Design review of the part shown in the three views and the two pictorial views. Dimensions are in mm from the part's minimum x, y and z. A direction names the side the tool comes from. Coordinates: 2 decimals unless noted, no trailing zeros. Loops run counter-clockwise (first coordinate to the right, second up) from the corner with the lowest first, then second, coordinate; pieces in that order, holes last. Notation, with made-up numbers: (4.25, -26.5) -> (19.25, -26.5) arc R22 cw to (19.25, 1.5) -> close; hole circle Ø9 at (78, 37.5). An arc over 180 degrees is marked (long way). One line per item, written item: value. Start each with the question number.
1. Add section D-D on y = 3.5. Write out the cut boundary in (x, z).
2. Insertion check: pin 1 (1.1 mm diameter, centred on x = 8.5, z = 1.5, fed in from -Y); pin 2 (4 mm diameter, centred on x = 16, y = 4, fed in from +Z). Each pin has a flat end and moves straight along its axis. Give the tip position at first contact, or say it passes through.
3. For probe 1 along Y at (x, z) = (5.25, 1.75); probe 2 along Z at (x, y) = (12, 3.5); probe 3 along Y at (x, z) = (4.5, 8.75), list the stretches that pass through material, from the lowest coordinate up.
4. Add section A-A on y = 1.75. Write out the cut boundary in (x, z).
5. Machinability: for the marked faces 1 and 2, which of the approach directions +Z, -Z, +X, -X, +Y, -Y give a long, thin tool a straight path to every point of the face, cutting with its end or side? Answer none if there is none.
6. Add section C-C on x = 11. Write out the cut boundary in (y, z).
7. Add section B-B on z = 2.5. Write out the cut boundary in (x, y).
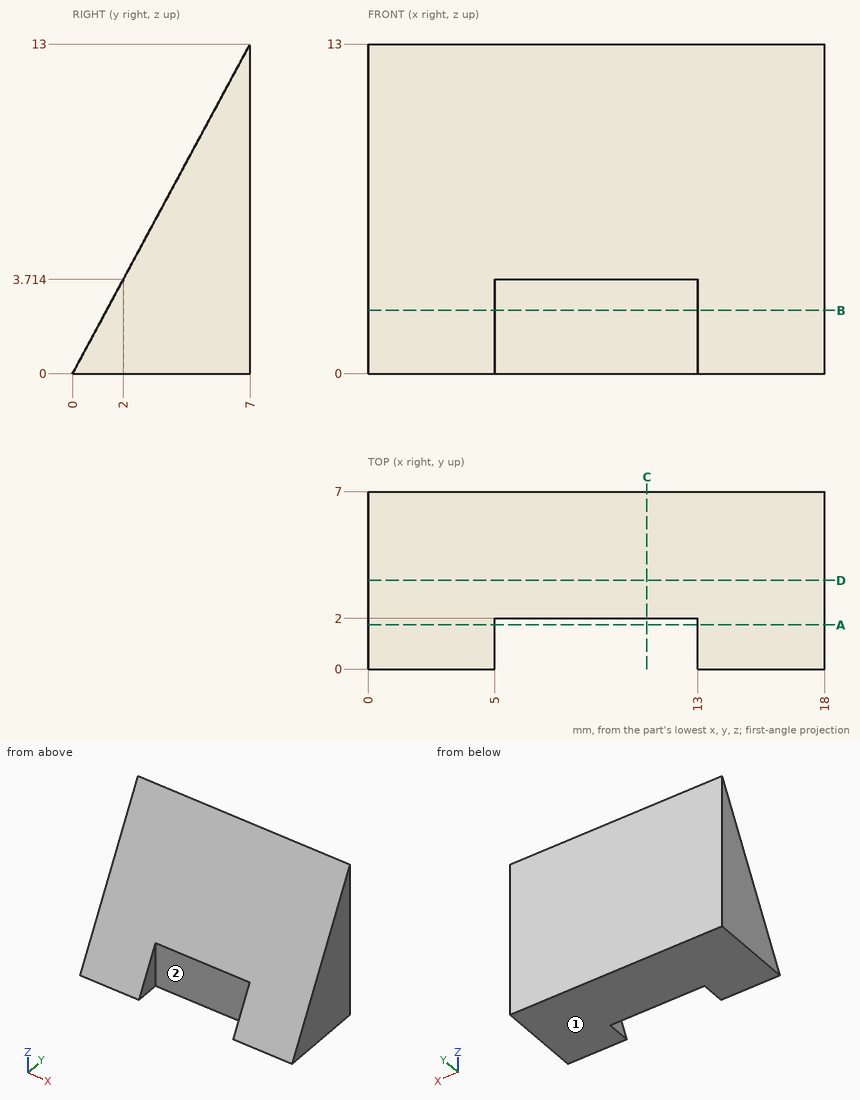
Worked answers:
1. outline: (0, 0) -> (18, 0) -> (18, 6.5) -> (0, 6.5) -> close
2. pin 1: stops at y = 2
2. pin 2: stops at z = 11.14
3. probe 1: y = 2 to 7
3. probe 2: z = 0 to 6.5
3. probe 3: y = 4.71 to 7
4. outline: (0, 0) -> (5, 0) -> (5, 3.25) -> (0, 3.25) -> close; (13, 0) -> (18, 0) -> (18, 3.25) -> (13, 3.25) -> close
5. face 1: -Z, +X, -X, +Y, -Y
5. face 2: +Z, -Z, -Y
6. outline: (2, 0) -> (7, 0) -> (7, 13) -> (2, 3.71) -> close
7. outline: (0, 1.35) -> (5, 1.35) -> (5, 2) -> (13, 2) -> (13, 1.35) -> (18, 1.35) -> (18, 7) -> (0, 7) -> close
